Answer from the drawing. Dimensions are ordinates in mm from the lowest x, y and z of the part. A direction names the side the tool comes from. Coordinates: 2 decimals unless noted, no trailing zeros. Order: outer loops, then holes, each group sorted by start corner. A loop starts at its lowest first (then second) coordinate and runs counter-clockwise, first axis right, second up. Notation, with made-up numbers: (5, 39) -> (25, 39) arc R9 cw to (25, 48) -> close; hole circle Ø5 at (2, -39). An arc over 180 degrees is marked (long way). Answer as a JSON object with one key per item and string values. Group by question number.
1) Given pin 1 (2 mm diameter, centred on x = 6, y = 13.5, fed in from -Z); pin 2 (1 mm diameter, centred on x = 10.5, y = 8.5, fed in from +Z), each flat-ended and moving along its own axis, determine where each tip first touches the part or whether it passes through.
2) Determine the mould class of the marked faces 3 and 4 for opening direction X: released by +X, released by -X, zero draft, split by the parting line, or undercut.
3) Section C-C on z = 2.9 is taken. Determine the outline of the cut face in (x, y), and give its area (3 significant figures).
4) A tool of negligible diameter and unlimited length cuts with its end or side. For the marked faces 1 and 2, from which of +Z, -Z, +X, -X, +Y, -Y can it reach the whole face along a straight path? Write none if from no direction.
5) Consider L1, parallel to Y at x = 8, z = 0.35; L2, parallel to Y at x = 8, z = 0.25; L3, parallel to Y at x = 8, z = 1.85. Determine where each line is inside the solid, lowest interval first.
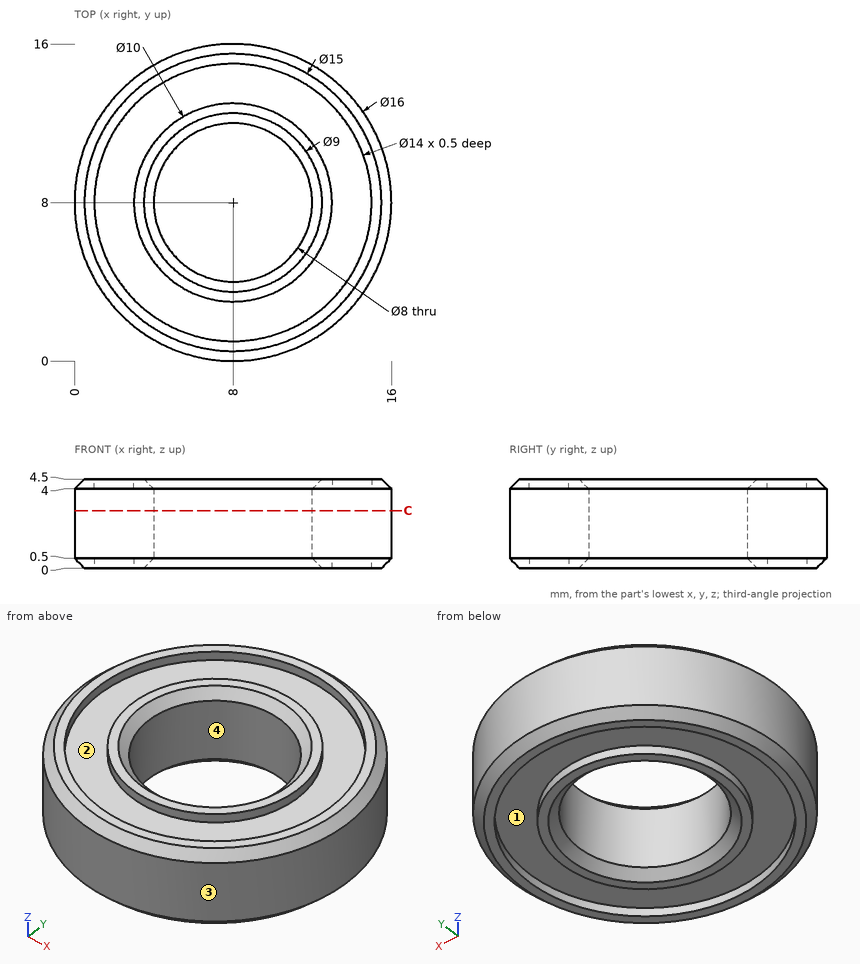
Worked answers:
{
 "1": {"pin 1": "stops at z = 0", "pin 2": "passes through"},
 "2": {"face 3": "split by the parting line", "face 4": "undercut"},
 "3": {"outline": "circle Ø16 at (8, 8); hole circle Ø8 at (8, 8)", "area": "151 mm²"},
 "4": {"face 1": "-Z", "face 2": "+Z"},
 "5": {"L1": "y = 0.15 to 1, 3 to 3.85, 12.15 to 13, 15 to 15.85", "L2": "y = 0.25 to 1, 3 to 3.75, 12.25 to 13, 15 to 15.75", "L3": "y = 0 to 4, 12 to 16"}
}
